Could you check a few things on this model? Use its own coordinates, in mm. A direction names the side the tool comes from. Coordinates: 2 decimals unless noted, no trailing zeros. Write each loop counter-clockwise with the first axis right and the second up, starting at its lowest first coordinate (ties: lowest second). Pieces come first, ordered by that corner, then holes.
Autodesk Inventor part; units mm, degrees
ref_plane "YZ Plane" through (0, 0, 0) normal (1, 0, 0) x (0, 1, 0)
ref_plane "XZ Plane" through (0, 0, 0) normal (0, 1, 0) x (-1, 0, 0)
ref_plane "XY Plane" through (0, 0, 0) normal (0, 0, 1) x (1, 0, 0)
sketch "スケッチ1" plane through (0, 0, 0) normal (0, 0, 1) x (1, 0, 0)
  circle A0 centre (0, 0) radius 4
  dimension "d0" = 8
extrude "押し出し1" add sketch "スケッチ1" along normal blind 65
sketch "スケッチ2" plane through (0, 0, 65) normal (0, 0, 1) x (1, 0, 0)
  point P0 (0, 0)
  point P1 (0, 0)
hole "穴1" at (0, 0, 65) direction (0, 0, -1) diameter 2.459 depth 8.8 tip angle 118
sketch "スケッチ3" plane through (0, 0, 0) normal (0, 0, -1) x (-1, 0, 0)
  circle A0 centre (0, 0) radius 1.2295
hole "穴2" at (0, 0, 0) direction (0, 0, 1) diameter 2.459 depth 8.8 tip angle 118
properties part number "link1part4" material "アルミニウム 6061"
Item 1: I want a section at B-B, the plane z = 23. List the corners of the cut face in (x, y) for me.
Item 2: Which directions (+Z, -Z, +X, -X, +Y, -Y) give clear straight access to the entire face, cutting with the end or side of a thin tool? Please do faces 5 (the flat face through (-1, -1, 0)), 6 (the cylindrical face through (0.748, 0.976, 60.538)).
Item 3: I want a section at C-C, the plane x = -3. List the corners of the cut face in (y, z) for me.
Item 4: Will these pins go through, and if not, where does the flat tip stop? pin 1 Ø3 at (y, z) = (-2.5, 46) entering from +X; pin 2 Ø4 at (x, z) = (2, 26.5) entering from -Y; pin 3 Ø2 at (x, y) = (0, 0) entering from +Z; pin 4 Ø2 at (y, z) = (-3, 46.5) entering from -X.
Item 5: I want a section at D-D, the plane y = 2. List the corners of the cut face in (x, z) for me, then the cut area to 3 significant figures.
Item 6: I want a section at A-A, the plane z = 6. List the corners of the cut face in (x, y) for me.
Item 7: If I drill on line 1 along Y through (x, z) = (0, 62.5); line 2 along X through (y, z) = (-0.75, 57); line 3 along X through (y, z) = (-3.5, 55), over which ranges is the centre line in solid material (lowest first)?
Item 8: If we mould it in two halves opening along Y, with no side actions, what happens to faces 1 (the conical face through (0.064, 0.204, 9.41)), 2 (the cylindrical face through (-0.867, 3.905, 32.045)), 3 (the flat face through (-1, -1, 65)), 4 (the cylindrical face through (0.748, -0.976, 4.462))? For each: released by +Y, released by -Y, zero draft, split by the parting line, or undercut.
Taken from the geometry:
1. outline: circle Ø8 at (0, 0)
2. face 5: -Z, +X, -X, +Y, -Y
2. face 6: +Z
3. outline: (-2.65, 0) - (2.65, 0) - (2.65, 65) - (-2.65, 65) - close
4. pin 1: stops at x = 3.87
4. pin 2: stops at y = -4
4. pin 3: stops at z = 56.06
4. pin 4: stops at x = -3.46
5. outline: (-3.46, 0) - (3.46, 0) - (3.46, 65) - (-3.46, 65) - close
5. area: 450 mm2
6. outline: circle Ø8 at (0, 0); hole circle Ø2.46 at (0, 0)
7. line 1: y = -4 to -1.23, 1.23 to 4
7. line 2: x = -3.93 to -0.97, 0.97 to 3.93
7. line 3: x = -1.94 to 1.94
8. face 1: undercut
8. face 2: split by the parting line
8. face 3: zero draft
8. face 4: undercut
